```python
from build123d import *

# Parameters (mm, degrees)
F1_DEPTH = 50
F3_D     = 5
F3_DEPTH = 30
F4_R     = 4.159464
F4_R_2   = 2.5
F4_R_3   = 4.212355
F5_DEPTH = 2.5


with BuildPart() as f1:
    # F0 (on Front) → F1 (new body)
    with BuildSketch(Plane.XZ):
        Polygon((-74.577573, 9.925295), (-62.995659, 9.925295), (-62.995659, 12.425295), (-62.995659, 14.925295), (-74.577573, 14.925295), align=None)
        Polygon((-62.995659, 29.925295), (-74.577573, 29.925295), (-74.577573, 24.925295), (-62.995659, 24.925295), (-62.995659, 27.425295), align=None)
        Polygon((-49.536098, 27.425295), (-54.305424, 27.425295), (-54.23216, 26.4727), (-53.230801, 25.296023), (-51.729051, 24.932656), (-50.300528, 25.521392), (-49.490879, 26.837354), align=None)
        Polygon((-14.193381, 29.925295), (-62.995659, 29.925295), (-62.995659, 27.425295), (-54.305424, 27.425295), (-54.350643, 28.013235), (-53.540994, 29.329197), (-52.112471, 29.917933), (-50.610722, 29.554566), (-49.609363, 28.37789), (-49.536098, 27.425295), (-44.420761, 27.425295), (-43.943304, 28.894758), (-42.693304, 29.802936), (-41.148219, 29.802936), (-39.898219, 28.894758), (-39.420761, 27.425295), (-34.420761, 27.425295), (-33.943304, 28.894758), (-32.693304, 29.802936), (-31.148219, 29.802936), (-29.898219, 28.894758), (-29.420761, 27.425295), (-24.420761, 27.425295), (-23.943304, 28.894758), (-22.693304, 29.802936), (-21.148219, 29.802936), (-19.898219, 28.894758), (-19.420761, 27.425295), (-14.193381, 27.425295), align=None)
        Polygon((-54.350643, 28.013235), (-54.305424, 27.425295), (-49.536098, 27.425295), (-49.609363, 28.37789), (-50.610722, 29.554566), (-52.112471, 29.917933), (-53.540994, 29.329197), align=None)
        Polygon((-43.943304, 28.894758), (-44.420761, 27.425295), (-39.420761, 27.425295), (-39.898219, 28.894758), (-41.148219, 29.802936), (-42.693304, 29.802936), align=None)
        Polygon((-39.420761, 27.425295), (-44.420761, 27.425295), (-43.943304, 25.955832), (-42.693304, 25.047653), (-41.148219, 25.047653), (-39.898219, 25.955832), align=None)
        Polygon((-29.898219, 25.955832), (-29.420761, 27.425295), (-34.420761, 27.425295), (-33.943304, 25.955832), (-32.693304, 25.047653), (-31.148219, 25.047653), align=None)
        Polygon((-34.420761, 27.425295), (-29.420761, 27.425295), (-29.898219, 28.894758), (-31.148219, 29.802936), (-32.693304, 29.802936), (-33.943304, 28.894758), align=None)
        Polygon((-24.420761, 27.425295), (-19.420761, 27.425295), (-19.898219, 28.894758), (-21.148219, 29.802936), (-22.693304, 29.802936), (-23.943304, 28.894758), align=None)
        Polygon((-19.898219, 25.955832), (-19.420761, 27.425295), (-24.420761, 27.425295), (-23.943304, 25.955832), (-22.693304, 25.047653), (-21.148219, 25.047653), align=None)
        Polygon((-54.036331, 13.757347), (-54.3733, 12.425295), (-49.468223, 12.425295), (-49.426269, 12.591143), (-50.000157, 14.025695), (-51.307652, 14.848948), (-52.849333, 14.746448), align=None)
        Polygon((-49.468223, 12.425295), (-54.3733, 12.425295), (-54.415254, 12.259447), (-53.841365, 10.824895), (-52.533871, 10.001641), (-50.99219, 10.104141), (-49.805191, 11.093243), align=None)
        Polygon((-44.383395, 12.425295), (-39.458127, 12.425295), (-39.42397, 12.551915), (-39.97524, 13.99531), (-41.269633, 14.839012), (-42.812735, 14.760757), (-44.015134, 13.790434), align=None)
        Polygon((-39.826389, 11.060155), (-39.458127, 12.425295), (-44.383395, 12.425295), (-44.417553, 12.298674), (-43.866282, 10.85528), (-42.571889, 10.011577), (-41.028787, 10.089833), align=None)
        Polygon((-34.370867, 12.425295), (-29.470655, 12.425295), (-29.799939, 13.748969), (-30.983016, 14.742758), (-32.52428, 14.851354), (-33.83502, 14.033279), (-34.414579, 12.601008), align=None)
        Polygon((-29.426944, 12.249582), (-29.470655, 12.425295), (-34.370867, 12.425295), (-34.041583, 11.10162), (-32.858506, 10.107832), (-31.317242, 9.999235), (-30.006502, 10.817311), align=None)
        Polygon((-24.31116, 12.425295), (-19.530363, 12.425295), (-19.635516, 13.439028), (-20.667817, 14.588655), (-22.1787, 14.911953), (-23.591059, 14.285431), (-24.365421, 12.9484), align=None)
        Polygon((-19.476102, 11.902189), (-19.530363, 12.425295), (-24.31116, 12.425295), (-24.206006, 11.411561), (-23.173706, 10.261934), (-21.662823, 9.938637), (-20.250464, 10.565158), align=None)
        Polygon((-14.193381, 9.925295), (-14.193381, 12.425295), (-19.530363, 12.425295), (-19.476102, 11.902189), (-20.250464, 10.565158), (-21.662823, 9.938637), (-23.173706, 10.261934), (-24.206006, 11.411561), (-24.31116, 12.425295), (-29.470655, 12.425295), (-29.426944, 12.249582), (-30.006502, 10.817311), (-31.317242, 9.999235), (-32.858506, 10.107832), (-34.041583, 11.10162), (-34.370867, 12.425295), (-39.458127, 12.425295), (-39.826389, 11.060155), (-41.028787, 10.089833), (-42.571889, 10.011577), (-43.866282, 10.85528), (-44.417553, 12.298674), (-44.383395, 12.425295), (-49.468223, 12.425295), (-49.805191, 11.093243), (-50.99219, 10.104141), (-52.533871, 10.001641), (-53.841365, 10.824895), (-54.415254, 12.259447), (-54.3733, 12.425295), (-62.995659, 12.425295), (-62.995659, 9.925295), align=None)
        Polygon((-9.193381, 29.925295), (-14.193381, 29.925295), (-14.193381, 27.425295), (-14.193381, 12.425295), (-14.193381, 9.925295), (-9.193381, 9.925295), (-9.193381, 11.774359), (-9.193381, 25.814013), (-9.193381, 27.425295), align=None)
        Polygon((48.476379, 29.925295), (-9.193381, 29.925295), (-9.193381, 27.425295), (42.382944, 27.425295), (48.476379, 27.425295), align=None)
        Polygon((16.594782, 19.599827), (-9.193381, 27.425295), (-9.193381, 25.814013), (13.939861, 18.794186), align=None)
        Polygon((48.476379, 27.425295), (42.382944, 27.425295), (16.594782, 19.599827), (13.939861, 18.794186), (-9.193381, 11.774359), (-9.193381, 9.925295), align=None)
    extrude(amount=F1_DEPTH)

    # F3
    with Locations(Plane.XY.offset(29.925295)):
        with Locations((-69.248043, -11.523538), (-69.248043, -36.80516)):
            Hole(F3_D / 2, depth=F3_DEPTH)

    # F4 (on face) → F5 (cut)
    with BuildSketch(Plane.XY.offset(29.925295)):
        with Locations((-69.248043, -11.523538)):
            Circle(F4_R)
        with Locations((-69.248043, -11.523538)):
            Circle(F4_R_2, mode=Mode.SUBTRACT)
        with Locations((-69.248043, -36.80516)):
            Circle(F4_R_3)
        with Locations((-69.248043, -36.80516)):
            Circle(F4_R_2, mode=Mode.SUBTRACT)
    extrude(amount=-F5_DEPTH, mode=Mode.SUBTRACT)


solid = f1.part
```
CAD build for the part. Positions are in the model's coordinates, mm. A direction names the side the tool comes from. Round coordinates to 2 decimals unless told otherwise and drop trailing zeros. Order: outer loops, then holes, each group sorted by start corner. A loop starts at its lowest first (then second) coordinate and runs counter-clockwise, first axis right, second up. Notation, with made-up numbers: (-24.5, 85.25) - (28.5, 85.25) arc R21 cw to (28.5, 91.25) - close; hole circle Ø6 at (6.5, 77.5). An arc over 180 degrees is marked (long way). Use CSV: the item, a comma, the result in double quotes. Start each with the question number.
1) Wall check: L1, parallel to Z at x = -49, y = -16; L2, parallel to Z at x = -4.5, y = -15; L3, parallel to Z at x = 3.5, y = -25. Give the ranges that are in metal, low to high. Write a range as [from, to].
2) Saw through at B-B (z = 22.75). List the corners of the cut face in (x, y), and give its area (3 significant figures).
3) Two-plate mould, pull along Y, no slides. Class faces 4 (the flat face through (-67, -13, 27.425)), 5 (the flat face through (-47, -25, 12.425)): pulls with the +Y half, pulls with the -Y half, needs draft (parallel to the pull), parting line crosses it, or undercut.
4) Saw through at A-A (x = -36). List the corners of the cut face in (y, z), and give its area (3 significant figures).
5) Saw through at D-D (x = 34.5). List the corners of the cut face in (y, z), and give its area (3 significant figures).
6) Pin check, flat tips, straight feed: pin 1 Ø25 at (x, y) = (19.5, -16) entering from -Z; pin 2 Ø6 at (x, y) = (-69.25, -36.81) entering from +Z. Stop position of each tip, or through.
7) Saw through at C-C (y = -31.5). Count the separate pieces of the cut face and the enclosed holes in it, and give its area (3 significant figures).
8) Tool access for faces 1 (the cylindrical face through (-65.4, -13.1, 28.7)), 2 (the flat face through (-17, -25, 12.425)), 3 (the flat face through (-12, -25, 29.925)): list every direction of +Z, -Z, +X, -X, +Y, -Y with a clear straight run to the whole face (end or side of a thin tool).
Values follow:
1,L1,"z = [9.93, 12.43], [27.43, 29.93]"
1,L2,"z = [11.35, 13.2], [24.39, 26], [27.43, 29.93]"
1,L3,"z = [13.78, 15.63], [21.96, 23.57], [27.43, 29.93]"
2,outline,"(-14.19, -50) - (-9.19, -50) - (-9.19, 0) - (-14.19, 0) - close; (0.9, -50) - (6.21, -50) - (6.21, 0) - (0.9, 0) - close; (26.98, -50) - (33.07, -50) - (33.07, 0) - (26.98, 0) - close"
2,area,"820 mm2"
3,face 4,"undercut"
3,face 5,"needs draft"
4,outline,"(-50, 9.93) - (0, 9.93) - (0, 12.43) - (-50, 12.43) - close; (-50, 27.43) - (0, 27.43) - (0, 29.93) - (-50, 29.93) - close"
4,area,"250 mm2"
5,outline,"(-50, 23.18) - (0, 23.18) - (0, 25.03) - (-50, 25.03) - close; (-50, 27.43) - (0, 27.43) - (0, 29.93) - (-50, 29.93) - close"
5,area,"217 mm2"
6,pin 1,"stops at z = 14.84"
6,pin 2,"stops at z = 27.43"
7,separate pieces,"1"
7,enclosed holes,"2"
7,area,"818 mm2"
8,face 1,"+Z"
8,face 2,"+Y, -Y"
8,face 3,"+Z, +X, -X, +Y, -Y"
